For this review, take the finished solid that the model builds, in its own axes (mm). A direction names the side the tool comes from. Round coordinates to 2 decimals unless told otherwise and drop trailing zeros. Order: outer loops, then holes, each group sorted by start corner. A loop starts at its lowest first (then second) coordinate and runs counter-clockwise, first axis right, second up. Notation, with made-up numbers: (47, 20) - (104, 20) arc R23 cw to (104, 46) - close; hole circle Ø2 at (-28.5, 19). An arc over 180 degrees is marked (long way). Write each question's results on one line, items separated by ' | '. Start each with the question number.
(1) Take a section at C-C, the plane y = -4. Give the boundary of the cut face in (x, z).
(2) For faces 5 (the flat face through (-17, -2.564, 7)), 6 (the flat face through (-36, 15.769, 7)), 7 (the flat face through (8, 11, 5)), list the 3-axis set-ups (+Z, -Z, +X, -X, +Y, -Y) from which the entire face can be reached by the end or side of a thin tool; tool diameter is ignored.
(3) Take a section at B-B, the plane z = 13.25. Give the boundary of the cut face in (x, y).
(4) Insertion check: pin 1 Ø3.5 at (x, z) = (-38.5, 9.5) entering from -Y; pin 2 Ø8 at (x, z) = (-56, 7.5) entering from +Y; pin 3 Ø6 at (y, z) = (26.5, 3.5) entering from +X. Each pin has a flat end and moves straight along its axis. Give the tip position at first contact, or say it passes through.
(5) Draft analysis for pull direction Y (two halves, no side actions). For faces 1 (the cylindrical face through (10.3, 14, 2.5)), 2 (the cylindrical face through (18.28, 0.82, 10.07)), 3 (the cylindrical face through (-66.953, 11.099, 7.395)), 4 (the flat face through (-18, 11, 15)), state which applies: pulls with the +Y half, pulls with the -Y half, needs draft (parallel to the pull), parting line crosses it, or undercut.
(6) Take a section at A-A, the plane y = 13.5. Give the boundary of the cut face in (x, z), plus the area to 3 significant figures.
(7) For L1, parallel to X at y = 12, z = 6.25; L2, parallel to Y at x = -31, z = 2.75; L3, parallel to Y at x = -28, z = 11, list the stretches that pass through material, from the lowest coordinate up. Write a range as from..to.
(8) Take a section at D-D, the plane x = -16.5. Give the boundary of the cut face in (y, z).
```python
from build123d import *

# Parameters (mm, degrees)
BOSS_EXTRUDE3_DEPTH = 15
SKETCH5_R           = 11.1
CUT_EXTRUDE2_DEPTH  = 10
SKETCH8_R           = 5
CUT_EXTRUDE5_DEPTH  = 10
SKETCH10_R          = 7.5
SKETCH10_W          = 12
SKETCH10_H          = 10.5
CUT_EXTRUDE6_DEPTH  = 16


with BuildPart() as part:
    # Sketch4 → Boss-Extrude3 (new body)
    with BuildSketch(Plane.XY):
        with BuildLine():
            Line((-31.83399024, -2.564162853), (-1.83399024, -2.564162853))
            ThreePointArc((-1.83399024, -2.564162853), (33.162534063, 10.767212745), (-1.964197709, 23.75162662))
            Line((-1.964197709, 23.75162662), (-31.964197709, 23.75162662))
            ThreePointArc((-31.964197709, 23.75162662), (-66.960722012, 10.420251021), (-31.83399024, -2.564162853))
        make_face()
    extrude(amount=BOSS_EXTRUDE3_DEPTH)

    # Sketch5 → Cut-Extrude2 (cut)
    with BuildSketch(Plane.XY.offset(15)):
        with Locations((13.162778875, 10.66825628)):
            Circle(SKETCH5_R)
    extrude(amount=-CUT_EXTRUDE2_DEPTH, mode=Mode.SUBTRACT)

    # Sketch8 → Cut-Extrude5 (cut)
    with BuildSketch(Plane.XY.offset(5)):
        with Locations((14.03064546, 10.66825628)):
            Circle(SKETCH8_R)
    extrude(amount=-CUT_EXTRUDE5_DEPTH, mode=Mode.SUBTRACT)

    # Sketch10 → Cut-Extrude6 (cut, through all)
    with BuildSketch(Plane(origin=(0, 0, 0), x_dir=(-1, 0, 0), z_dir=(0, 0, -1))):
        with Locations((46.960966823, 10.519207486)):
            Circle(SKETCH10_R)
        with Locations((36.330902029, 10.519207486)):
            Rectangle(SKETCH10_W, SKETCH10_H)
    extrude(amount=-CUT_EXTRUDE6_DEPTH, mode=Mode.SUBTRACT)


solid = part.part
```
Results below:
1) outline: (-60.72, 0) - (-33.21, 0) - (-33.21, 15) - (-60.72, 15) - close; (-0.43, 0) - (26.76, 0) - (26.76, 15) - (-0.43, 15) - close
2) face 5: +Z, -Z, -Y | face 6: +Z, -Z | face 7: +Z
3) outline: (-31.96, 23.75) arc R20 ccw (long way) to (-31.83, -2.56) - (-1.83, -2.56) arc R20 ccw (long way) to (-1.96, 23.75) - close; hole (-41.6, 5.27) - (-30.33, 5.27) - (-30.33, 15.77) - (-41.6, 15.77) arc R7.5 ccw (long way) to start; hole circle Ø22.2 at (13.16, 10.67)
4) pin 1: stops at y = -8.32 | pin 2: stops at y = 29.87 | pin 3: stops at x = 28.5
5) face 1: undercut | face 2: undercut | face 3: parting line crosses it | face 4: needs draft
6) outline: (-66.74, 0) - (-53.84, 0) - (-53.84, 15) - (-66.74, 15) - close; (-30.33, 0) - (9.91, 0) - (9.91, 5) - (2.43, 5) - (2.43, 15) - (-30.33, 15) - close; (18.15, 0) - (32.96, 0) - (32.96, 15) - (23.9, 15) - (23.9, 5) - (18.15, 5) - close | area: 887 mm^2
7) L1: x = -66.91..-54.31, -30.33..2.14, 24.18..33.12 | L2: y = -2.56..5.27, 15.77..23.75 | L3: y = -2.56..23.75
8) outline: (-2.56, 0) - (23.75, 0) - (23.75, 15) - (-2.56, 15) - close
